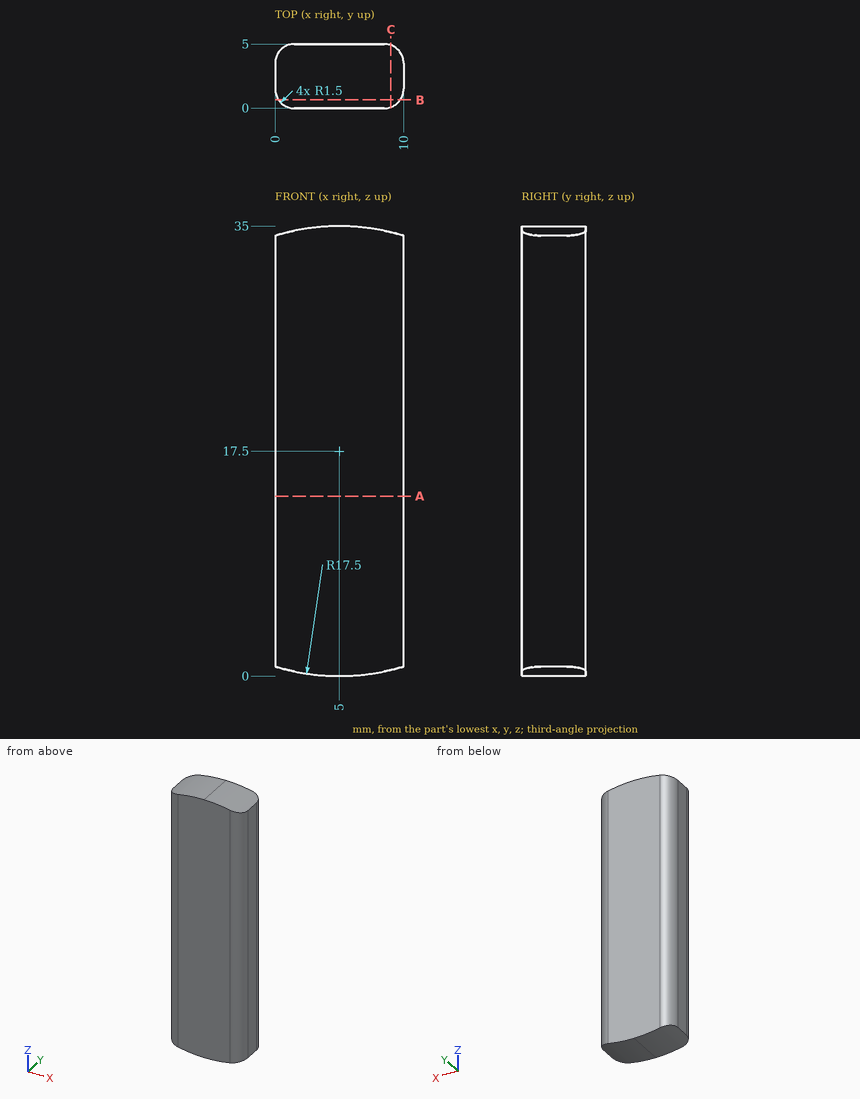
Geometry check sheet. Reference: drawing and pictorial views, mm from the part's lowest x, y, z. Give positions to 0.01 mm unless a question says otherwise; leave off trailing zeros. Order: outer loops, then holes, each group sorted by start corner. A loop starts at its lowest first (then second) coordinate and runs counter-clockwise, first axis right, second up.
1. Thickness scan on L1, parallel to Z at x = 4.5, y = 4.2; L2, parallel to X at y = 1.4, z = 22; L3, parallel to Y at x = 1, z = 9.5. Record the ranges inside material, lowest first.
2. Section check A-A, the plane z = 14. Enter the section's corners in (x, y).
3. Section check B-B, the plane y = 0.65. Enter the section's corners in (x, z), and give its area (3 significant figures).
4. Section check C-C, the plane x = 9. Enter the section's corners in (y, z).
5. Gauge pin test, flat ends, axial feed: pin 1 Ø1 at (x, y) = (8.5, 3) entering from -Z; pin 2 Ø1.5 at (x, y) = (2, 4) entering from +Z; pin 3 Ø1.5 at (x, y) = (7.5, 3.5) entering from -Z. Record the tip position at first contact, or that the pin passes through.
Values follow:
1. L1: z = 0.01 to 34.99
1. L2: x = 0 to 10
1. L3: y = 0.09 to 4.91
2. outline: (0, 1.5) arc R1.5 ccw to (1.5, 0) - (8.5, 0) arc R1.5 ccw to (10, 1.5) - (10, 3.5) arc R1.5 ccw to (8.5, 5) - (1.5, 5) arc R1.5 ccw to (0, 3.5) - close
3. outline: (0.26, 0.65) arc R17.5 ccw to (9.74, 0.65) - (9.74, 34.35) arc R17.5 ccw to (0.26, 34.35) - close
3. area: 327 mm2
4. outline: (0.09, 0.46) - (4.91, 0.46) - (4.91, 34.54) - (0.09, 34.54) - close
5. pin 1: stops at z = 0.26
5. pin 2: stops at z = 34.85
5. pin 3: stops at z = 0.09
